The listing builds one solid part. Answer for the finished solid, in the listing's coordinates (mm). A direction names the side the tool comes from. Coordinates: 2 decimals unless noted, no trailing zeros. Write each loop counter-clockwise with the first axis right and the second up, starting at its lowest first coordinate (ties: lowest second). Pieces come first, ordered by that corner, then holes.
from build123d import *

# Parameters (mm, degrees)
BOSS_EXTRUDE1_DEPTH = 4.85
FILLET1_R           = 5
FILLET2_R           = 40
FILLET3_R           = 5
CHAMFER1_SIZE       = 1
CHAMFER2_SIZE       = 1
CHAMFER3_SIZE       = 1
BOSS_EXTRUDE2_START = -9.7
BOSS_EXTRUDE2_DEPTH = 9.7
CHAMFER4_SIZE       = 1


with BuildPart() as part:
    # Sketch1 → Boss-Extrude1 (new, symmetric)
    with BuildSketch(Plane.XY):
        Polygon((4.85, 55), (21.213203436, 38.636796564), (25.455844123, 42.879437252), (8.485281374, 59.85), (25.455844123, 76.820562748), (21.213203436, 81.063203436), (-4.85, 55), (-4.85, -55), (4.85, -55), align=None)
    extrude(amount=BOSS_EXTRUDE1_DEPTH, both=True)

    # Fillet1
    fillet1_edges = [part.edges().sort_by_distance(p)[0] for p in [
        (4.85, 55, 0),
    ]]
    fillet(fillet1_edges, radius=FILLET1_R)

    # Fillet2
    fillet2_edges = [part.edges().sort_by_distance(p)[0] for p in [
        (-4.85, 55, 0),
    ]]
    fillet(fillet2_edges, radius=FILLET2_R)

    # Fillet3
    fillet3_edges = [part.edges().sort_by_distance(p)[0] for p in [
        (8.485281374, 59.85, 0),
    ]]
    fillet(fillet3_edges, radius=FILLET3_R)

    # Chamfer1
    chamfer1_edges = [part.edges().sort_by_distance(p)[0] for p in [
        (21.213203436, 81.063203436, 0),
        (25.455844123, 76.820562748, 0),
        (25.455844123, 42.879437252, 0),
        (21.213203436, 38.636796564, 0),
    ]]
    chamfer(chamfer1_edges, length=CHAMFER1_SIZE)

    # Chamfer2
    # the kernel refuses this chamfer: 1 mm, written as the material it takes off along each edge
    with BuildSketch(Plane(origin=(-4.85, 38.431457505, -4.85), x_dir=(0.9996219169112968, 0, -0.027495876610586487), z_dir=(0, -1, 0)), Plane(origin=(-4.85, 38.431457505, 4.85), x_dir=(-0.027495876610586487, 0, -0.9996219169112968), z_dir=(0, -1, 0))) as chamfer2_piece_1:
        Polygon((CHAMFER2_SIZE * 0.999621916911, CHAMFER2_SIZE * 0.0274958766106), (-CHAMFER2_SIZE * 0.0274958766106, CHAMFER2_SIZE * 0.999621916911), (0, 0), align=None)
    extrude(amount=96.003140493, mode=Mode.SUBTRACT)
    with BuildSketch(Plane(origin=(35.15, 38.431457505, -4.85), x_dir=(-1, 0, 0), z_dir=(0, -1, 0))) as chamfer2_piece_2:
        Polygon((40 - CHAMFER2_SIZE, 0), (40, -CHAMFER2_SIZE), (40, 0), align=None)
    revolve(axis=Axis((35.15, 38.431457505, -4.85), (0, 0, -1)), revolution_arc=45, mode=Mode.SUBTRACT)
    with BuildSketch(Plane(origin=(22.324551134, 82.174551134, -4.85), x_dir=(0.7068394360706736, -0.7068394360706733, -0.027495876610586494), z_dir=(-0.7071067811865475, -0.7071067811865477, 0)), Plane(origin=(22.324551134, 82.174551134, 4.85), x_dir=(-0.019442520806010343, 0.019442520806010336, -0.999621916911297), z_dir=(-0.7071067811865475, -0.7071067811865477, 0))) as chamfer2_piece_3:
        Polygon((CHAMFER2_SIZE * 0.999621916911, CHAMFER2_SIZE * 0.0274958766106), (-CHAMFER2_SIZE * 0.0274958766106, CHAMFER2_SIZE * 0.999621916911), (0, 0), align=None)
    extrude(amount=21.862076271, mode=Mode.SUBTRACT)
    with BuildSketch(Plane(origin=(26.567191821, 75.70921505, -4.85), x_dir=(-0.7068394360706752, -0.7068394360706718, -0.02749587661058676), z_dir=(-0.7071067811865458, 0.7071067811865493, 0)), Plane(origin=(26.567191821, 75.70921505, 4.85), x_dir=(0.019442520806010388, 0.019442520806010295, -0.999621916911297), z_dir=(-0.7071067811865458, 0.7071067811865493, 0)), Plane(origin=(20.101855737, 37.525448866, -4.85), x_dir=(-0.7068394360706738, 0.7068394360706732, -0.027495876610586494), z_dir=(0.7071067811865472, 0.7071067811865478, 0)), Plane(origin=(20.101855737, 37.525448866, 4.85), x_dir=(0.019442520806015523, -0.01944252080601551, -0.9996219169112968), z_dir=(0.7071067811865472, 0.7071067811865478, 0))) as chamfer2_piece_4:
        Polygon((CHAMFER2_SIZE * 0.999621916911, CHAMFER2_SIZE * 0.0274958766106), (-CHAMFER2_SIZE * 0.0274958766106, CHAMFER2_SIZE * 0.999621916911), (0, 0), align=None)
    extrude(amount=9.143365976, mode=Mode.SUBTRACT)
    with BuildSketch(Plane(origin=(35.15, 38.431457505, 4.85), x_dir=(-1, 0, 0), z_dir=(0, -1, 0))) as chamfer2_piece_5:
        Polygon((40, CHAMFER2_SIZE), (40 - CHAMFER2_SIZE, 0), (40, 0), align=None)
    revolve(axis=Axis((35.15, 38.431457505, 4.85), (0, 0, -1)), revolution_arc=45, mode=Mode.SUBTRACT)
    with BuildSketch(Plane(origin=(12.02081528, 63.385533906, 4.85), x_dir=(0.019442520806015513, -0.01944252080601552, -0.9996219169112968), z_dir=(0.7071067811865476, 0.7071067811865475, 0)), Plane(origin=(26.567191821, 41.768089553, 4.85), x_dir=(0.019442520806015516, 0.019442520806015516, -0.9996219169112968), z_dir=(-0.7071067811865476, 0.7071067811865476, 0)), Plane(origin=(12.02081528, 63.385533906, -4.85), x_dir=(-0.7068394360706736, 0.7068394360706736, -0.027495876610586462), z_dir=(0.7071067811865476, 0.7071067811865475, 0)), Plane(origin=(26.567191821, 41.768089553, -4.85), x_dir=(-0.7068394360706735, -0.7068394360706735, -0.027495876610586494), z_dir=(-0.7071067811865476, 0.7071067811865476, 0))) as chamfer2_piece_6:
        Polygon((CHAMFER2_SIZE * 0.999621916911, CHAMFER2_SIZE * 0.0274958766106), (-CHAMFER2_SIZE * 0.0274958766106, CHAMFER2_SIZE * 0.999621916911), (0, 0), align=None)
    extrude(amount=20.571682988, mode=Mode.SUBTRACT)
    with BuildSketch(Plane(origin=(15.556349186, 59.85, 4.85), x_dir=(-0.7071067811865474, 0.7071067811865477, 0), z_dir=(0.7071067811865477, 0.7071067811865474, 0))) as chamfer2_piece_7:
        Polygon((5, -CHAMFER2_SIZE), (5 + CHAMFER2_SIZE, 0), (5, 0), align=None)
    revolve(axis=Axis((15.556349186, 59.85, 4.85), (0, 0, 1)), revolution_arc=90, mode=Mode.SUBTRACT)
    with BuildSketch(Plane(origin=(15.556349186, 59.85, -4.85), x_dir=(-0.7071067811865474, 0.7071067811865477, 0), z_dir=(0.7071067811865477, 0.7071067811865474, 0))) as chamfer2_piece_8:
        Polygon((5 + CHAMFER2_SIZE, 0), (5, CHAMFER2_SIZE), (5, 0), align=None)
    revolve(axis=Axis((15.556349186, 59.85, -4.85), (0, 0, 1)), revolution_arc=90, mode=Mode.SUBTRACT)
    with BuildSketch(Plane(origin=(13.385533906, 46.464466094, -4.85), x_dir=(0.7068394360706735, 0.7068394360706737, -0.027495876610586462), z_dir=(0.7071067811865477, -0.7071067811865474, 0)), Plane(origin=(13.385533906, 46.464466094, 4.85), x_dir=(-0.019442520806016373, -0.01944252080601638, -0.9996219169112965), z_dir=(0.7071067811865477, -0.7071067811865474, 0))) as chamfer2_piece_9:
        Polygon((CHAMFER2_SIZE * 0.999621916911, CHAMFER2_SIZE * 0.0274958766106), (-CHAMFER2_SIZE * 0.0274958766106, CHAMFER2_SIZE * 0.999621916911), (0, 0), align=None)
    extrude(amount=12.641679399, mode=Mode.SUBTRACT)
    with BuildSketch(Plane(origin=(9.85, 42.928932188, -4.85), x_dir=(0.7071067811865479, 0.7071067811865471, 0), z_dir=(0.7071067811865471, -0.7071067811865479, 0))) as chamfer2_piece_10:
        Polygon((5 + CHAMFER2_SIZE, 0), (5, CHAMFER2_SIZE), (5, 0), align=None)
    revolve(axis=Axis((9.85, 42.928932188, -4.85), (0, 0, 1)), revolution_arc=135, mode=Mode.SUBTRACT)
    with BuildSketch(Plane(origin=(4.85, -57.571682988, -4.85), x_dir=(-0.9996219169112968, 0, -0.027495876610586487), z_dir=(0, 1, 0)), Plane(origin=(4.85, -57.571682988, 4.85), x_dir=(0.027495876610586487, 0, -0.9996219169112968), z_dir=(0, 1, 0))) as chamfer2_piece_11:
        Polygon((CHAMFER2_SIZE * 0.999621916911, CHAMFER2_SIZE * 0.0274958766106), (-CHAMFER2_SIZE * 0.0274958766106, CHAMFER2_SIZE * 0.999621916911), (0, 0), align=None)
    extrude(amount=100.500615176, mode=Mode.SUBTRACT)
    with BuildSketch(Plane(origin=(9.85, 42.928932188, 4.85), x_dir=(0.7071067811865479, 0.7071067811865471, 0), z_dir=(0.7071067811865471, -0.7071067811865479, 0))) as chamfer2_piece_12:
        Polygon((5, -CHAMFER2_SIZE), (5 + CHAMFER2_SIZE, 0), (5, 0), align=None)
    revolve(axis=Axis((9.85, 42.928932188, 4.85), (0, 0, 1)), revolution_arc=135, mode=Mode.SUBTRACT)

    # Chamfer3
    # the kernel refuses this chamfer: 1 mm, written as the material it takes off along each edge
    with BuildSketch(Plane(origin=(4.85, -55, 6.421682988), x_dir=(-0.9996219169112968, -0.027495876610589075, 0), z_dir=(0, 0, -1)), Plane(origin=(-6.421682988, -55, 4.85), x_dir=(0, -0.02749587661058907, -0.9996219169112965), z_dir=(1, 0, 0)), Plane(origin=(-6.421682988, -55, -4.85), x_dir=(0, 0.9996219169112968, -0.027495876610586414), z_dir=(1, 0, 0))) as chamfer3_piece_1:
        Polygon((CHAMFER3_SIZE * 0.999621916911, CHAMFER3_SIZE * 0.0274958766106), (-CHAMFER3_SIZE * 0.0274958766106, CHAMFER3_SIZE * 0.999621916911), (0, 0), align=None)
    extrude(amount=12.843365976, mode=Mode.SUBTRACT)
    with BuildSketch(Plane(origin=(-4.85, -55, 6.421682988), x_dir=(0.9996219169112968, -0.027495876610589075, 0), z_dir=(0, 0, -1))) as chamfer3_piece_2:
        Polygon((CHAMFER3_SIZE * 0.999621916911, -CHAMFER3_SIZE * 0.0274958766106), (-CHAMFER3_SIZE * 0.0274958766106, -CHAMFER3_SIZE * 0.999621916911), (0, 0), align=None)
    extrude(amount=12.843365976, mode=Mode.SUBTRACT)

    # Sketch2 → Boss-Extrude2 (add)
    with BuildSketch(Plane.XY.offset(4.85).offset(BOSS_EXTRUDE2_START)):
        Polygon((-3.85, 5), (-9.85, 5), (-9.85, 8), (-3.85, 14), align=None)
    extrude(amount=BOSS_EXTRUDE2_DEPTH)

    # Chamfer4
    chamfer4_edges = [part.edges().sort_by_distance(p)[0] for p in [
        (-6.85, 11, 4.85),
        (-9.85, 6.5, 4.85),
        (-6.85, 5, 4.85),
        (-6.85, 11, -4.85),
        (-9.85, 6.5, -4.85),
        (-6.85, 5, -4.85),
        (-9.85, 5, 0),
    ]]
    chamfer(chamfer4_edges, length=CHAMFER4_SIZE)


solid = part.part
Q1. Which of the six approach directions +Z, -Z, +X, -X, +Y, -Y give full straight-line access (tool end or side, diameter ignored) to faces 1 (the face through (17.419, 43.128, 4.343)), 2 (the face through (16.9, 42.95, 0.05)), 3 (the face through (18.12, 70.18, 4.34)), 4 (the face through (-7, 5, 0))?
Answers below:
face 1: +Z, -Y
face 2: +Z, -Z, -Y
face 3: +Z, +X
face 4: +Z, -Z, -X, -Y
Q2. The part is cut by section A-A, the plane z = 2.5. Write down the section's boundary in (x, y).
Answers below:
outline: (-9.85, 6) - (-8.85, 5) - (-4.85, 5) - (-4.85, -54) - (-3.85, -55) - (3.85, -55) - (4.85, -54) - (4.85, 42.93) arc R5 cw to (13.39, 46.46) - (20.51, 39.34) - (21.92, 39.34) - (24.75, 42.17) - (24.75, 43.59) - (12.02, 56.31) arc R5 cw to (12.02, 63.39) - (24.75, 76.11) - (24.75, 77.53) - (21.92, 80.36) - (20.51, 80.36) - (6.87, 66.72) arc R40 ccw to (-4.85, 38.43) - (-4.85, 13) - (-9.85, 8) - close
Q3. The part is cut by section C-C, the plane x = -6.5. Write down the section's boundary in (y, z).
Answers below:
outline: (5, -3.85) - (6, -4.85) - (9.94, -4.85) - (11.35, -3.85) - (11.35, 3.85) - (9.94, 4.85) - (6, 4.85) - (5, 3.85) - close
Q4. Find the intervals of material crossed by probe 1 along X at (y, z) = (-15, 0.25); probe 2 along Y at (x, z) = (17.5, -2.75), in increasing order.
Answers below:
probe 1: x = -4.85 to 4.85
probe 2: y = 42.35 to 50.84, 68.86 to 77.35
Q5. Given pin 1 (1.5 mm diameter, centred on y = 56.5, z = -1, fed in from -X); pin 2 (2.5 mm diameter, centred on y = -25.5, z = 0, fed in from -X); pin 3 (4.5 mm diameter, centred on x = -7, z = 0.5, fed in from -Y); pin 4 (1 mm diameter, centred on x = 5.5, y = -38.5, fed in from -Z), each flat-ended and moving along its own axis, determine where each tip first touches the part or whether it passes through.
Answers below:
pin 1: stops at x = -0.91
pin 2: stops at x = -4.85
pin 3: stops at y = -54.1
pin 4: passes through
Q6. The part is cut by section B-B, the plane y = 1.5. Write down the section's boundary in (x, z), then the cut area to 3 significant figures.
Answers below:
outline: (-4.85, -3.85) - (-3.85, -4.85) - (3.85, -4.85) - (4.85, -3.85) - (4.85, 3.85) - (3.85, 4.85) - (-3.85, 4.85) - (-4.85, 3.85) - close
area: 92.1 mm2
